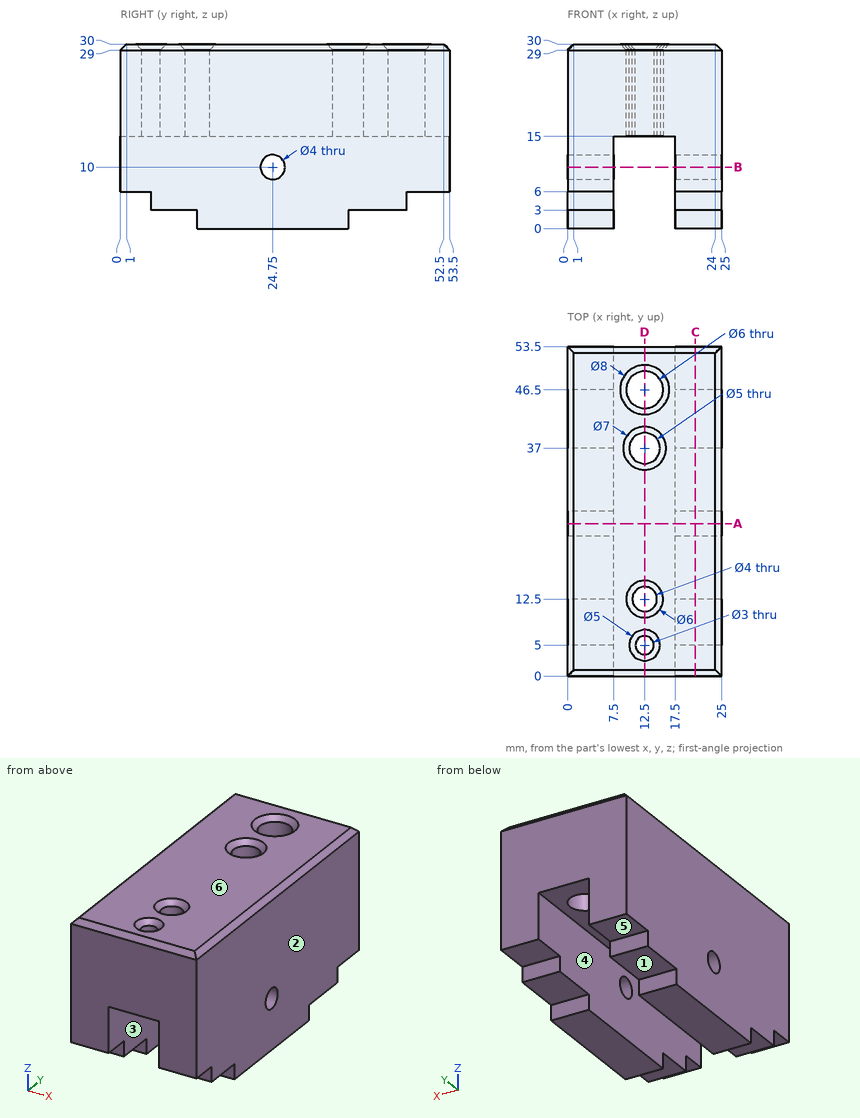
Answer from the drawing. Dimensions are ordinates in mm from the lowest x, y and z of the part. A direction names the side the tool comes from. Give positions to 0.01 mm unless a question says otherwise; leave off trailing zeros. Write each loop counter-clockwise with the first axis right and the second up, starting at its lowest first coordinate (ties: lowest second). Pieces come first, ordered by that corner, then holes. Notation, with made-up numbers: (-35.75, -31) - (-23.75, -31) arc R29 ccw to (-23.75, -11) - close; hole circle Ø9 at (52.5, 14.5). An arc over 180 degrees is marked (long way). One line per item, written item: value. Start each with the question number.
1. Given pin 1 (4 mm diameter, centred on x = 12.5, y = 37, fed in from +Z); pin 2 (0.9 mm diameter, centred on x = 21, z = 5, fed in from +Y); pin 3 (0.9 mm diameter, centred on x = 20, z = 4.5, fed in from -Y); pin 4 (3.5 mm diameter, centred on x = 4.5, z = 4.5, fed in from +Y), each flat-ended and moving along its own axis, determine where each tip first touches the part or whether it passes through.
2. Find section A-A (y = 24.75). Write down the section's boundary in (x, z).
3. Find section D-D (x = 12.5). State how many separate pieces and enclosed holes the cut face has, then the cut area to 4 significant figures.
4. Find section C-C (x = 20.75). Write down the section's boundary in (y, z), then the cut area to 3 significant figures.
5. Consider probe 1 along Y at (x, z) = (12.5, 26); probe 2 along Z at (x, y) = (6, 24.75); probe 3 along X at (y, z) = (44.5, 13). Determine where each line is inside the solid, lowest interval first.
6. For a pull along X with two mould halves and no side action, classify the marked faces 1, 2 and 3 as +X half, -X half, draft (parallel to the pull), parting line (faces both ways), or undercut.
7. Find section B-B (z = 10). Write down the section's boundary in (x, y).
8. For the marked faces 4, 5 and 6, determine the directions among +Z, -Z, +X, -X, +Y, -Y from which every point of the face is accessible in a straight line to the end or side of a thin tool.
Geometry results:
1. pin 1: through
1. pin 2: y = 46.5
1. pin 3: y = 5
1. pin 4: y = 53.5
2. outline: (0, 0) - (7.5, 0) - (7.5, 8) - (0, 8) - close; (0, 12) - (7.5, 12) - (7.5, 15) - (17.5, 15) - (17.5, 12) - (25, 12) - (25, 29) - (24, 30) - (1, 30) - (0, 29) - close; (17.5, 0) - (25, 0) - (25, 8) - (17.5, 8) - close
3. separate pieces: 5
3. enclosed holes: 0
3. area: 527.5 mm2
4. outline: (0, 6) - (5, 6) - (5, 3) - (12.5, 3) - (12.5, 0) - (37, 0) - (37, 3) - (46.5, 3) - (46.5, 6) - (53.5, 6) - (53.5, 29) - (52.5, 30) - (1, 30) - (0, 29) - close; hole circle Ø4 at (24.75, 10)
4. area: 1,470 mm2
5. probe 1: 0 to 3.5, 6.5 to 10.5, 14.5 to 34.5, 39.5 to 43.5, 49.5 to 53.5
5. probe 2: 0 to 8, 12 to 30
5. probe 3: 0 to 7.5, 17.5 to 25
6. face 1: draft
6. face 2: +X half
6. face 3: undercut
7. outline: (0, 0) - (7.5, 0) - (7.5, 22.75) - (0, 22.75) - close; (0, 26.75) - (7.5, 26.75) - (7.5, 53.5) - (0, 53.5) - close; (17.5, 0) - (25, 0) - (25, 22.75) - (17.5, 22.75) - close; (17.5, 26.75) - (25, 26.75) - (25, 53.5) - (17.5, 53.5) - close
8. face 4: -Z, +Y, -Y
8. face 5: -Z, +X, -X, +Y
8. face 6: +Z, +X, -X, +Y, -Y
